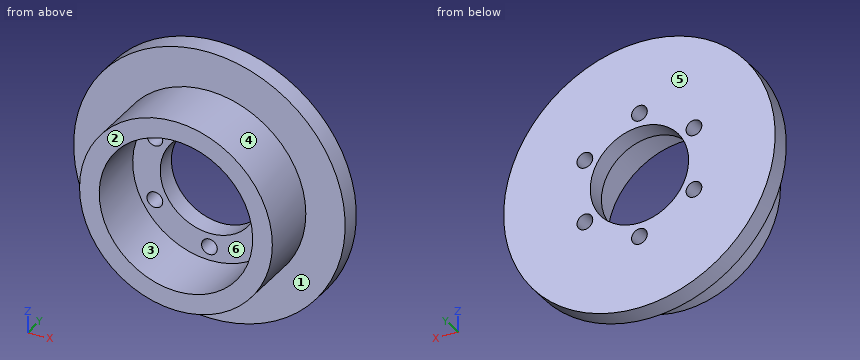
```python
from build123d import *

# Parameters (mm, degrees)
CROQUIS1_R              = 34.5
SALIENTE_EXTRUIR1_DEPTH = 5
CROQUIS2_R              = 24.5
CROQUIS2_R_2            = 19.5
SALIENTE_EXTRUIR2_DEPTH = 15
CROQUIS5_R              = 12.5
CORTAR_EXTRUIR2_DEPTH   = 52.044098582
CROQUIS7_R              = 2
CORTAR_EXTRUIR3_DEPTH   = 52.044098582
MATRIZC1_COUNT          = 6


with BuildPart() as part:
    # Croquis1 → Saliente-Extruir1 (new body)
    with BuildSketch(Plane(origin=(0, 0, 0), x_dir=(1, 0, 0), z_dir=(0, 1, 0))):
        with Locations(Location((0, 0, 0), (0, 0, 270))):
            Circle(CROQUIS1_R)
    extrude(amount=SALIENTE_EXTRUIR1_DEPTH)

    # Croquis2 → Saliente-Extruir2 (add)
    with BuildSketch(Plane.XZ):
        with Locations(Location((0, 0, 0), (0, 0, 90))):
            Circle(CROQUIS2_R)
        with Locations(Location((0, 0, 0), (0, 0, 270))):
            Circle(CROQUIS2_R_2, mode=Mode.SUBTRACT)
    extrude(amount=SALIENTE_EXTRUIR2_DEPTH)

    # Croquis5 → Cortar-Extruir2 (cut, through all)
    with BuildSketch(Plane.XZ):
        with Locations(Location((0, 0, 0), (0, 0, 270))):
            Circle(CROQUIS5_R)
    extrude(amount=-CORTAR_EXTRUIR2_DEPTH, mode=Mode.SUBTRACT)

    # Croquis7 → Cortar-Extruir3 (cut, through all)
    with BuildSketch(Plane.XZ):
        with Locations(Location((0, -16, 0), (0, 0, 270))):
            Circle(CROQUIS7_R)
    cortar_extruir3 = extrude(amount=-CORTAR_EXTRUIR3_DEPTH, mode=Mode.SUBTRACT)

    # MatrizC1: Cortar-Extruir3 ×6 about axis
    matrizc1_axis = Axis((0, 0, 0), (0, 1, 0))
    for i in range(1, MATRIZC1_COUNT):
        add(cortar_extruir3.rotate(matrizc1_axis, i * 360 / MATRIZC1_COUNT), mode=Mode.SUBTRACT)


solid = part.part
```
Can you work these out from the model? Positions are in its coordinate system, mm. Face numbers are marked on the shaded views. A direction names the side the tool comes from. Round coordinates to 2 decimals unless told otherwise and drop trailing zeros. Order: outer loops, then holes, each group sorted by start corner. A loop starts at its lowest first (then second) coordinate and runs counter-clockwise, first axis right, second up.
(1) If we section it at D-D (z = -8): Please give me the cut outline in (x, y), plus the area to 3 significant figures.
Results are:
outline: (-33.56, 0) - (-23.16, 0) - (-23.16, -15) - (-17.78, -15) - (-17.78, 0) - (-15.86, 0) - (-15.86, 5) - (-33.56, 5) - close; (-11.86, 0) - (-9.6, 0) - (-9.6, 5) - (-11.86, 5) - close; (9.6, 0) - (11.86, 0) - (11.86, 5) - (9.6, 5) - close; (15.86, 0) - (17.78, 0) - (17.78, -15) - (23.16, -15) - (23.16, 0) - (33.56, 0) - (33.56, 5) - (15.86, 5) - close
area: 361 mm2
(2) If I drill on L1, parallel to X at y = 0.5, z = 8; L2, parallel to Y at x = 7, z = 28; L3, parallel to Z at x = 1.5, y = -13.5, over which ranges is the centre line in solid material (lowest first)?
Results are:
L1: x = -33.56 to -15.86, -11.86 to -9.6, 9.6 to 11.86, 15.86 to 33.56
L2: y = 0 to 5
L3: z = -24.45 to -19.44, 19.44 to 24.45
(3) I'm going to push flat-ended pins straight in: pin 1 (2 mm diameter, centred on x = 7.5, y = -2.5, fed in from -Z); pin 2 (1 mm diameter, centred on x = -5.5, y = -4.5, fed in from -Z); pin 3 (6.5 mm diameter, centred on x = 0, z = -16, fed in from -Y); pin 4 (19.5 mm diameter, centred on x = 2, z = 1, fed in from -Y). Where does each tip first touch, or does it pass through?
Results are:
pin 1: stops at z = -23.62
pin 2: stops at z = -23.98
pin 3: stops at y = 0
pin 4: passes through
(4) If we section it at C-C (x = 14.5): Please give me the cut outline in (y, z).
Results are:
outline: (-15, -19.75) - (0, -19.75) - (0, -31.3) - (5, -31.3) - (5, -9.89) - (0, -9.89) - (0, -13.04) - (-15, -13.04) - close; (-15, 13.04) - (0, 13.04) - (0, 9.89) - (5, 9.89) - (5, 31.3) - (0, 31.3) - (0, 19.75) - (-15, 19.75) - close; (0, -6.11) - (5, -6.11) - (5, 6.11) - (0, 6.11) - close
(5) We'd pull the mould along Z, two halves only. Please class the marked faces 3, 4, 5 and 6: +Z half, -Z half, draft (parallel to the pull), parting line (faces both ways), or undercut.
Results are:
face 3: undercut
face 4: parting line
face 5: draft
face 6: undercut
(6) If we section it at A-A (x = 0): Please give me the cut outline in (y, z), plus the area to 3 significant figures.
Results are:
outline: (-15, -24.5) - (0, -24.5) - (0, -34.5) - (5, -34.5) - (5, -18) - (0, -18) - (0, -19.5) - (-15, -19.5) - close; (-15, 19.5) - (0, 19.5) - (0, 18) - (5, 18) - (5, 34.5) - (0, 34.5) - (0, 24.5) - (-15, 24.5) - close; (0, -14) - (5, -14) - (5, -12.5) - (0, -12.5) - close; (0, 12.5) - (5, 12.5) - (5, 14) - (0, 14) - close
area: 330 mm2
(7) On a 3-axis mill with a long thin cutter (end or side, diameter ignored), from which of +Z, -Z, +X, -X, +Y, -Y can I reach the whole of each face in a straight line? I mean the marked faces 1 and 2. Say none if no direction works.
Results are:
face 1: -Y
face 2: +Z, -Z, +X, -X, -Y
(8) If we section it at B-B (z = 0): Please give me the cut outline in (x, y), plus the area to 3 significant figures.
Results are:
outline: (-34.5, 0) - (-24.5, 0) - (-24.5, -15) - (-19.5, -15) - (-19.5, 0) - (-12.5, 0) - (-12.5, 5) - (-34.5, 5) - close; (12.5, 0) - (19.5, 0) - (19.5, -15) - (24.5, -15) - (24.5, 0) - (34.5, 0) - (34.5, 5) - (12.5, 5) - close
area: 370 mm2
